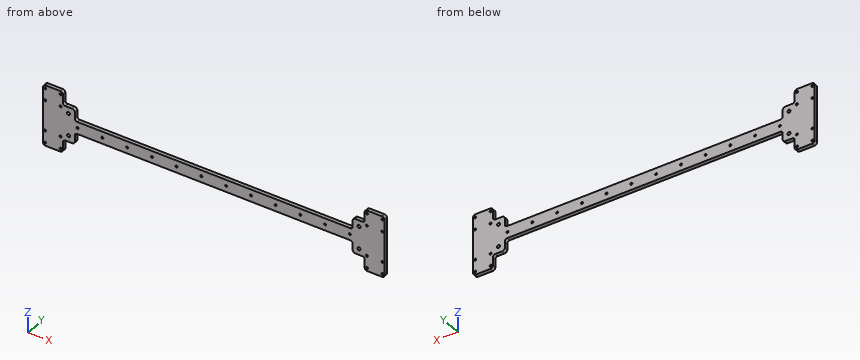
```python
from build123d import *

# Parameters (mm, degrees)
SKETCH1_W            = 552
SKETCH1_H            = 20
BOSS_EXTRUDE1_DEPTH  = 6
SKETCH3_W            = 32
SKETCH3_H            = 100
BOSS_EXTRUDE2_DEPTH  = 6
M3_CLEARANCE_HOLE1_D = 3.4
SKETCH10_W           = 19.392395665
SKETCH10_H           = 18.526197832
SKETCH10_R           = 2.525
BOSS_EXTRUDE3_DEPTH  = 6
FILLET2_R            = 4
FILLET2_OF_MIRROR1_R = 4


with BuildPart() as part:
    # Sketch1 → Boss-Extrude1 (new body)
    with BuildSketch(Plane(origin=(0, 0, 0), x_dir=(1, 0, 0), z_dir=(0, 1, 0))):
        with Locations((276, 10)):
            Rectangle(SKETCH1_W, SKETCH1_H)
    extrude(amount=BOSS_EXTRUDE1_DEPTH)

    # Sketch3 → Boss-Extrude2 (add)
    with BuildSketch(Plane.XZ):
        with Locations((16, -10)):
            Rectangle(SKETCH3_W, SKETCH3_H)
    boss_extrude2 = extrude(amount=-BOSS_EXTRUDE2_DEPTH)

    # M3 Clearance Hole1 (through all)
    with Locations(Plane(origin=(0, 6, 0), x_dir=(1, 0, 0), z_dir=(0, 1, 0))):
        with Locations((3.5, -35), (3.5, -15), (28.5, -15), (28.5, -35), (3.5, 55), (28.5, 55), (28.5, 35), (3.5, 35), (56, 10), (96, 10), (136, 10), (176, 10), (216, 10), (256, 10)):
            m3_clearance_hole1 = Hole(M3_CLEARANCE_HOLE1_D / 2)

    # Sketch10 → Boss-Extrude3 (add)
    with BuildSketch(Plane(origin=(0, 6, 0), x_dir=(1, 0, 0), z_dir=(0, 1, 0))):
        with Locations((41.696197833, -9.263098916)):
            Rectangle(SKETCH10_W, SKETCH10_H)
        with Locations((41.232395665, -8.366197832)):
            Circle(SKETCH10_R, mode=Mode.SUBTRACT)
        with Locations((41.696197833, 29.263098916)):
            Rectangle(SKETCH10_W, SKETCH10_H)
        with Locations((41.232395665, 28.366197832)):
            Circle(SKETCH10_R, mode=Mode.SUBTRACT)
    boss_extrude3 = extrude(amount=-BOSS_EXTRUDE3_DEPTH)

    # Fillet2
    fillet2_edges = [part.edges().sort_by_distance(p)[0] for p in [
        (32, 3, 18.526197832),
        (51.392395665, 3, 0),
        (51.392395665, 3, 18.526197832),
        (32, 3, -38.526197832),
        (51.392395665, 3, -38.526197832),
        (51.392395665, 3, -20),
        (0, 3, -60),
        (32, 3, 40),
        (0, 3, 40),
        (32, 3, -60),
    ]]
    fillet(fillet2_edges, radius=FILLET2_R)

    # Mirror1: Boss-Extrude2, M3 Clearance Hole1, Boss-Extrude3 across plane
    add(boss_extrude2.mirror(Plane(origin=(276, 0, 0), x_dir=(0, 0, 1), z_dir=(1, 0, 0))))
    add(m3_clearance_hole1.mirror(Plane(origin=(276, 0, 0), x_dir=(0, 0, 1), z_dir=(1, 0, 0))), mode=Mode.SUBTRACT)
    add(boss_extrude3.mirror(Plane(origin=(276, 0, 0), x_dir=(0, 0, 1), z_dir=(1, 0, 0))))

    # Fillet2 of Mirror1
    fillet2_of_mirror1_edges = [part.edges().sort_by_distance(p)[0] for p in [
        (520, 3, 18.526197832),
        (500.607604335, 3, 0),
        (500.607604335, 3, 18.526197832),
        (520, 3, -38.526197832),
        (500.607604335, 3, -38.526197832),
        (500.607604335, 3, -20),
        (552, 3, -60),
        (520, 3, 40),
        (552, 3, 40),
        (520, 3, -60),
    ]]
    fillet(fillet2_of_mirror1_edges, radius=FILLET2_OF_MIRROR1_R)


solid = part.part
```
Source: CAD feature listing. Evaluate the final solid. Frame: model axes, mm. Coordinates: 2 decimals unless noted, no trailing zeros. Order: outer loops, then holes, each group sorted by start corner. A loop starts at its lowest first (then second) coordinate and runs counter-clockwise, first axis right, second up. Notation, with made-up numbers: (71.25, -36) - (90.25, -36) arc R6 cw to (90.25, -31) - close; hole circle Ø6 at (38.5, 13.5). An arc over 180 degrees is marked (long way). One line per item, written item: value.
1) Contact query for flat-ended pins moving along their axis: pin 1 (4 mm diameter, centred on x = 96, z = -10, fed in from -Y); pin 2 (3 mm diameter, centred on x = 41.5, y = 4, fed in from -Z); pin 3 (1 mm diameter, centred on x = 111, y = 4.5, fed in from +Z); pin 4 (2 mm diameter, centred on x = 337.5, y = 3, fed in from -Z). Output: stop coordinate, or through.
Computed values:
pin 1: stops at y = 0
pin 2: stops at z = -38.53
pin 3: stops at z = 0
pin 4: stops at z = -20
2) Cut plane B-B on y = 1.1. State how many separate pieces and enclosed holes the cut face has, plus the area to 3 significant figures.
Computed values:
separate pieces: 1
enclosed holes: 32
area: 17,200 mm^2
3) Cut plane A-A on x = 188. Output: boundary loops of the cut face in (y, z).
Computed values:
outline: (0, -20) - (6, -20) - (6, 0) - (0, 0) - close
4) Ray query, line 1 (X direction, y = 5, z = 9); line 2 (Z direction, x = 523.5, y = 4.6); line 3 (X direction, y = 0.95, z = 12.5). Return the intervals inside material, ascending. Write a range as [from, to].
Computed values:
line 1: x = [0, 38.79], [43.68, 51.39], [500.61, 508.32], [513.21, 552]
line 2: z = [-59.97, -56.7], [-53.3, -36.7], [-33.3, 13.3], [16.7, 33.3], [36.7, 39.97]
line 3: x = [0, 51.39], [500.61, 552]
